Model file for the job. Use its own axes, mm. Face numbers are marked on the shaded views. A direction names the side the tool comes from. Round coordinates to 2 decimals unless told otherwise and drop trailing zeros. Order: outer loops, then holes, each group sorted by start corner. A loop starts at its lowest first (then second) coordinate and runs counter-clockwise, first axis right, second up. Notation, with made-up numbers: (-38.5, 18.5) - (-24.5, 18.5) arc R30 cw to (-24.5, 51.5) - close; hole circle Ø2 at (20, 65). An arc over 180 degrees is marked (long way). Put each result on its own line as item: value. Start each with the question number.
Item 1: Mould opens along X. For the marked faces 6, 7 and 8 say: pulls with the +X half, pulls with the -X half, needs draft (parallel to the pull), parting line crosses it, or undercut.
Item 2: Pin check, flat tips, straight feed: pin 1 Ø5 at (y, z) = (-21, 220) entering from -X; pin 2 Ø2 at (y, z) = (-23, 215.5) entering from +X; pin 3 Ø1.5 at (x, z) = (10.5, 218) entering from +Y; pin 4 Ø1 at (y, z) = (-15.5, 224.5) entering from -X. Stop position of each tip, or through.
Item 3: Probe probe 1 along X at (y, z) = (-17.25, 217.25); probe 2 along Y at (x, z) = (0.5, 220.25); probe 3 along X at (y, z) = (-11.75, 214). List the from-to ranges inside material, lowest first.
Item 4: Saw through at A-A on y = -11.75. List the corners of the cut face in (x, z), plus the area to 3 significant figures.
Item 5: Saw through at B-B on y = -20. List the corners of the cut face in (x, z).
Item 6: Which spindle directions (+Z, -Z, +X, -X, +Y, -Y) get a long thin tool onto all of the face, cutting with end or side? Do the marked faces 1, 2, 3, 4 and 5. Say none if no direction does.
Item 7: Saw through at D-D on y = -15. List the corners of the cut face in (x, z), plus the area to 3 significant figures.
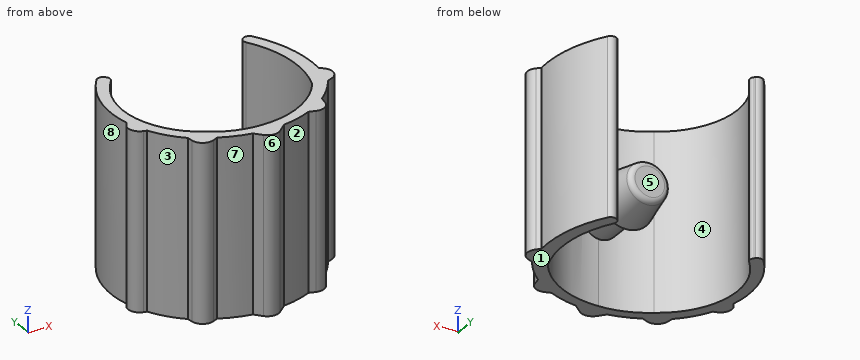
```python
from build123d import *

# Parameters (mm, degrees)
BOSS_EXTRUDE2_DEPTH      = 438
SCALE2_SCALE             = 0.0354
FILLET1_R                = 1
FILLET3_R                = 0.5
BOSS_EXTRUDE4_REACH      = 229.494
BOSS_EXTRUDE4_END_RADIUS = 7.833804904
BOSS_EXTRUDE5_REACH      = 229.494
BOSS_EXTRUDE5_END_RADIUS = 7.195916772
SKETCH9_R                = 2.45
BOSS_EXTRUDE6_DEPTH      = 3.5
BOSS_EXTRUDE6_TAPER      = 12
FILLET4_R                = 0.5


with BuildPart() as part:
    # Sketch1 → Boss-Extrude2 (new body)
    with BuildSketch(Plane.XY):
        with BuildLine():
            Line((-163.578194132, 204.291420663), (-186.376739015, 226.341062883))
            ThreePointArc((-186.376739015, 226.341062883), (-239.375206738, 127.519864833), (-240.870528276, 15.393905402))
            Line((-240.870528276, 15.393905402), (-268.785604462, -26.370002184))
            Line((-268.785604462, -26.370002184), (-221.583341967, -38.017313709))
            ThreePointArc((-221.583341967, -38.017313709), (-196.547148618, -77.434601057), (-164.251041881, -111.161370973))
            Line((-164.251041881, -111.161370973), (-156.910200465, -164.920829998))
            Line((-156.910200465, -164.920829998), (-109.836943046, -141.764303292))
            ThreePointArc((-109.836943046, -141.764303292), (-73.054639313, -155.90344513), (-34.693982777, -164.920829998))
            Line((-34.693982777, -164.920829998), (0, -203.328769621))
            Line((0, -203.328769621), (42.8865283, -164.920829998))
            ThreePointArc((42.8865283, -164.920829998), (80.850316946, -156.155814803), (117.057486625, -141.764303292))
            Line((117.057486625, -141.764303292), (163.626630073, -155.521102036))
            Line((163.626630073, -155.521102036), (172.334894528, -105.315261233))
            ThreePointArc((172.334894528, -105.315261233), (201.269995869, -76.001800701), (225.162074479, -42.450531906))
            Line((225.162074479, -42.450531906), (276.709162079, -20.095520822))
            Line((276.709162079, -20.095520822), (237.860130884, 17.793666683))
            ThreePointArc((237.860130884, 17.793666683), (228.121311005, 125.922470041), (181.39622554, 223.91965937))
            Line((181.39622554, 223.91965937), (156.421805868, 206.970503899))
            ThreePointArc((156.421805868, 206.970503899), (202.986661671, 88.666279899), (188.748912803, -37.672398736))
            ThreePointArc((188.748912803, -37.672398736), (107.904666904, -114.25255983), (0, -141.764303292))
            ThreePointArc((0, -141.764303292), (-60.71851518, -133.27976481), (-116.145688788, -107.077591147))
            ThreePointArc((-116.145688788, -107.077591147), (-216.983443781, 36.858584217), (-163.578194132, 204.291420663))
        make_face()
    extrude(amount=BOSS_EXTRUDE2_DEPTH)


with BuildPart() as part_1:
    # Scale2: scaled about (7.22089485, -18.85403102, 219)
    add(part.part.scale(SCALE2_SCALE).moved(Location((6.965275172, -18.186598322, 211.2474))))

    # Fillet1
    fillet1_edges = [part_1.edges().sort_by_distance(p)[0] for p in [
        (16.76077951, -18.897979759, 219),
        (12.757657877, -23.692045334, 219),
        (6.965275172, -25.384436766, 219),
        (1.410654076, -24.024795704, 219),
        (-2.549735226, -19.120096399, 219),
    ]]
    fillet(fillet1_edges, radius=FILLET1_R)

    # Fillet3
    fillet3_edges = [part_1.edges().sort_by_distance(p)[0] for p in [
        (12.5026071, -10.859842484, 219),
        (13.386701556, -10.25984238, 219),
        (0.367538611, -10.174124696, 219),
        (1.1746071, -10.95468203, 219),
    ]]
    fillet(fillet3_edges, radius=FILLET3_R)

    # Boss-Extrude4: up to this cylinder (the profile starts inside it)
    boss_extrude4_end = Plane(origin=(7.002032477, -15.371335991, 218.5826), z_dir=(0, 0, -1)) * Cylinder(BOSS_EXTRUDE4_END_RADIUS, 475.655609807, mode=Mode.PRIVATE)
    # Sketch5 → Boss-Extrude4 (add, up to the surface)
    with BuildSketch(Plane(origin=(0, -19.405054659, 0), x_dir=(-1, 0, 0), z_dir=(0, -1, 0)), mode=Mode.PRIVATE) as boss_extrude4_sk1:
        with BuildLine():
            Line((-6.838033993, -220.1826), (-6.838033993, -216.9826))
            ThreePointArc((-6.838033993, -216.9826), (-8.438033993, -218.5826), (-6.838033993, -220.1826))
        make_face()
    boss_extrude4_tool1 = extrude(boss_extrude4_sk1.sketch, amount=BOSS_EXTRUDE4_REACH, mode=Mode.PRIVATE) & boss_extrude4_end
    add(boss_extrude4_tool1.solids().sort_by_distance((7.517095, -19.405055, 218.5826))[0])

    # Boss-Extrude5: up to this cylinder (the profile starts inside it)
    boss_extrude5_end = Plane(origin=(6.875019163, -16.009703934, 218.5826), z_dir=(0, 0, -1)) * Cylinder(BOSS_EXTRUDE5_END_RADIUS, 474.379833545, mode=Mode.PRIVATE)
    # Sketch8 → Boss-Extrude5 (add, up to the surface)
    with BuildSketch(Plane(origin=(0, -19.405054659, 0), x_dir=(-1, 0, 0), z_dir=(0, -1, 0)), mode=Mode.PRIVATE) as boss_extrude5_sk1:
        with BuildLine():
            Line((-6.838033993, -216.9826), (-6.838033993, -220.1826))
            ThreePointArc((-6.838033993, -220.1826), (-5.238033993, -218.5826), (-6.838033993, -216.9826))
        make_face()
    boss_extrude5_tool1 = extrude(boss_extrude5_sk1.sketch, amount=BOSS_EXTRUDE5_REACH, mode=Mode.PRIVATE) & boss_extrude5_end
    add(boss_extrude5_tool1.solids().sort_by_distance((6.158973, -19.405055, 218.5826))[0])

    # Sketch9 → Boss-Extrude6 (add)
    with BuildSketch(Plane(origin=(0, -19.405054659, 0), x_dir=(1, 0, 0), z_dir=(0, 1, 0))):
        with Locations((6.838033993, -218.5826)):
            Circle(SKETCH9_R)
    extrude(amount=BOSS_EXTRUDE6_DEPTH, taper=BOSS_EXTRUDE6_TAPER)

    # Fillet4
    fillet4_edges = [part_1.edges().sort_by_distance(p)[0] for p in [
        (5.131981959, -15.905054659, 218.5826),
    ]]
    fillet(fillet4_edges, radius=FILLET4_R)


solid = part_1.part
```
Results found:
1. face 6: parting line crosses it
1. face 7: undercut
1. face 8: pulls with the -X half
2. pin 1: stops at x = -1.93
2. pin 2: stops at x = 13.05
2. pin 3: stops at y = -21.95
2. pin 4: stops at x = -1.77
3. probe 1: x = -1.64 to -0.65, 5.36 to 8.32, 14.18 to 15.41
3. probe 2: y = -21.5 to -19.89, -11.77 to -10.42
3. probe 3: x = -0.75 to 0.51, 13.06 to 14.28
4. outline: (-0.75, 211.25) - (0.51, 211.25) - (0.51, 226.75) - (-0.75, 226.75) - close; (13.06, 211.25) - (14.28, 211.25) - (14.28, 226.75) - (13.06, 226.75) - close
4. area: 38.5 mm²
5. outline: (-0.62, 211.25) - (0.58, 211.25) - (0.58, 226.75) - (-0.62, 226.75) - close; circle Ø3.2 at (6.84, 218.58); (13.32, 211.25) - (14.74, 211.25) - (14.74, 226.75) - (13.32, 226.75) - close
6. face 1: -Z, +X, -X, +Y, -Y
6. face 2: +Z, -Z, -Y
6. face 3: +Z, -Z, -X, -Y
6. face 4: +Z, -Z
6. face 5: +Z, -Z, +Y
7. outline: (-1.74, 211.25) - (-0.75, 211.25) - (-0.75, 226.75) - (-1.74, 226.75) - close; (14.14, 211.25) - (15.31, 211.25) - (15.31, 226.75) - (14.14, 226.75) - close
7. area: 33.4 mm²
